from build123d import *

# Parameters (mm, degrees)
PAD002_DEPTH         = 4
SKETCH012_R          = 11
POCKET008_DEPTH      = 4.001
POCKET008_DEPTH_BACK = 4.001
SKETCH023_R          = 2
POCKET015_DEPTH      = 209.948575
POCKET015_DEPTH_BACK = 209.948575
POLARPATTERN_COUNT   = 4


with BuildPart() as part:
    # Sketch011 → Pad002 (new body, symmetric)
    with BuildSketch(Plane.XY):
        with BuildLine():
            ThreePointArc((17.405807, -11.748953), (21, 0), (17.405807, 11.748953))
            Line((36.296696, 30.639841), (17.405807, 11.748953))
            ThreePointArc((36.296696, 30.639841), (33.587572, 33.587572), (30.639841, 36.296696))
            Line((11.748953, 17.405807), (30.639841, 36.296696))
            ThreePointArc((11.748953, 17.405807), (0, 21), (-11.748953, 17.405807))
            Line((-30.639841, 36.296696), (-11.748953, 17.405807))
            ThreePointArc((-30.639841, 36.296696), (-33.587572, 33.587572), (-36.296696, 30.639841))
            Line((-36.296696, 30.639841), (-17.405807, 11.748953))
            ThreePointArc((-17.405807, 11.748953), (-21, 0), (-17.405807, -11.748953))
            Line((-36.296696, -30.639841), (-17.405807, -11.748953))
            ThreePointArc((-36.296696, -30.639841), (-33.587572, -33.587572), (-30.639841, -36.296696))
            Line((-11.748953, -17.405807), (-30.639841, -36.296696))
            ThreePointArc((-11.748953, -17.405807), (0, -21), (11.748953, -17.405807))
            Line((11.748953, -17.405807), (30.639841, -36.296696))
            ThreePointArc((30.639841, -36.296696), (33.587572, -33.587572), (36.296696, -30.639841))
            Line((17.405807, -11.748953), (36.296696, -30.639841))
        make_face()
    extrude(amount=PAD002_DEPTH, both=True)

    # Sketch012 → Pocket008 (cut, two sides)
    with BuildSketch(Plane.XY) as pocket008_sk:
        Circle(SKETCH012_R)
    extrude(amount=-POCKET008_DEPTH, mode=Mode.SUBTRACT)
    extrude(pocket008_sk.sketch, amount=POCKET008_DEPTH_BACK, mode=Mode.SUBTRACT)

    # Sketch023 → Pocket015 (cut, two sides)
    with BuildSketch(Plane.XY) as pocket015_sk:
        with Locations((-31, 31)):
            Circle(SKETCH023_R)
    pocket015 = extrude(amount=-POCKET015_DEPTH, mode=Mode.SUBTRACT) + extrude(pocket015_sk.sketch, amount=POCKET015_DEPTH_BACK, mode=Mode.SUBTRACT)

    # PolarPattern: Pocket015 ×4 about axis
    polarpattern_axis = Axis((0, 0, 0), (0, 0, 1))
    for i in range(1, POLARPATTERN_COUNT):
        add(pocket015.rotate(polarpattern_axis, i * 360 / POLARPATTERN_COUNT), mode=Mode.SUBTRACT)


with BuildPart() as part_1:
    # Body005 placement: moved
    add(part.part.moved(Location((0, 0, 58))))


with BuildPart() as part_2:
    # Clone003 placement: moved
    add(part_1.part.moved(Location((0, 0, 20))))


with BuildPart() as part_3:
    # Body006 placement: moved
    add(part_2.part.moved(Location((0, 0, -136))))


solid = part_3.part
Verification items for the finished model (mm, model axes). A direction names the side the tool comes from. Coordinates: 2 decimals unless noted, no trailing zeros. Write each loop counter-clockwise with the first axis right and the second up, starting at its lowest first coordinate (ties: lowest second). Pieces come first, ordered by that corner, then holes. Notation, with made-up numbers: M 55.5,1.5 L 86.5,1.5 A11 ccw 86.5,20.5 Z; hole C 79.5,28.5 d6. An arc over 180 degrees is marked long. Use a Markdown table: item, result.
Q1. Set-up check for faces 1 (the face through (-21.062, -26.719, -57.944)), 2 (the face through (26.719, -21.062, -57.944)), 3 (the face through (-26.983, -21.327, -57.944)), 4 (the face through (-21.327, 26.983, -57.944)): record each of +Z, -Z, +X, -X, +Y, -Y from which the full face is reachable in a straight line by a thin tool's end or side.
Reply:
| item | result |
|---|---|
| face 1 | +Z, -Z, -Y |
| face 2 | +Z, -Z, +X |
| face 3 | +Z, -Z, -X |
| face 4 | +Z, -Z, +Y |
Q2. Thickness scan on line 1 (X direction, y = 0, z = -56.75); line 2 (Y direction, x = -31, z = -57.75). Record the ranges inside material, lowest first.
Reply:
| item | result |
|---|---|
| line 1 | x = -21 to -11, 11 to 21 |
| line 2 | y = -35.99 to -33, -29 to -25.34, 25.34 to 29, 33 to 35.99 |
Q3. Draft check along Y on faces 5 (the face through (3, 11, -54)), 6 (the face through (21.062, -26.719, -57.944)), 7 (the face through (-21, 0, -58)). Enter one of: +Y half, -Y half, draft (parallel to the pull), parting line (faces both ways), or undercut.
Reply:
| item | result |
|---|---|
| face 5 | draft |
| face 6 | -Y half |
| face 7 | undercut |
Q4. Sectioned sample at C-C, the plane z = -55.5. Record the boundary of the cut face in (x, y).
Reply:
| item | result |
|---|---|
| outline | M -36.3,-30.64 A47.5 ccw -30.64,-36.3 L -11.75,-17.41 A21 ccw 11.75,-17.41 L 30.64,-36.3 A47.5 ccw 36.3,-30.64 L 17.41,-11.75 A21 ccw 17.41,11.75 L 36.3,30.64 A47.5 ccw 30.64,36.3 L 11.75,17.41 A21 ccw -11.75,17.41 L -30.64,36.3 A47.5 ccw -36.3,30.64 L -17.41,11.75 A21 ccw -17.41,-11.75 Z; hole C -31,-31 d4; hole C -31,31 d4; hole C 0,0 d22; hole C 31,-31 d4; hole C 31,31 d4 |
Q5. Go/stop test with flat-tipped pins: P1, Ø13, axis at x = 0, y = 0, coming from the -Z side; P2, Ø2, axis at x = -17, z = -60, coming from the +Y side; P3, Ø1.5, axis at x = 22, z = -61, coming from the -Y side; P4, Ø4, axis at y = 0.5, z = -56.5, coming from the -X side. Record where each tip stops, or that it passes through.
Reply:
| item | result |
|---|---|
| P1 | passes through |
| P2 | stops at y = 23.66 |
| P3 | stops at y = -28.41 |
| P4 | stops at x = -21 |
Q6. Sectioned sample at A-A, the plane x = 0. Record the boundary of the cut face in (y, z).
Reply:
| item | result |
|---|---|
| outline | M -21,-62 L -11,-62 L -11,-54 L -21,-54 Z; M 11,-62 L 21,-62 L 21,-54 L 11,-54 Z |
